CAD build for the part. Positions are in the model's coordinates, mm. A direction names the side the tool comes from. Give positions to 0.01 mm unless a question says otherwise; leave off trailing zeros. Write each loop counter-clockwise with the first axis right and the second up, starting at its lowest first coordinate (ties: lowest second). Pieces come first, ordered by that corner, then holes. Notation, with made-up numbers: (-9, 2.5) -> (11, 2.5) arc R9 ccw to (11, 7.5) -> close; hole circle Ø1 at (-7, 85.5). An arc over 180 degrees is marked (long way). Use one line per item in the form item = value. Start each with the question number.
from build123d import *

# Parameters (mm, degrees)
SKETCH1_R           = 2.5
SKETCH1_R_2         = 4
BOSS_EXTRUDE1_DEPTH = 15
SKETCH2_R           = 6.5
CUT_EXTRUDE1_DEPTH  = 8
FILLET1_R           = 7.5
CUT_EXTRUDE2_DEPTH  = 5
SKETCH5_W           = 82.5
SKETCH5_H           = 15.853105066
CUT_EXTRUDE3_DEPTH  = 15
CUT_EXTRUDE4_DEPTH  = 5
SKETCH7_R           = 2.5
BOSS_EXTRUDE2_DEPTH = 0.4


with BuildPart() as part:
    # Sketch1 → Boss-Extrude1 (new body)
    with BuildSketch(Plane(origin=(0, 0, 0), x_dir=(1, 0, 0), z_dir=(0, 1, 0))):
        Polygon((39.925742574, 57.194719472), (57.425742574, 39.694719472), (57.425742574, -162.805280528), (-42.574257426, -162.805280528), (-42.574257426, 39.694719472), (-25.074257426, 57.194719472), align=None)
        with Locations((42.175742574, 43.694719472)):
            Circle(SKETCH1_R, mode=Mode.SUBTRACT)
        with Locations((-27.324257426, 43.694719472)):
            Circle(SKETCH1_R, mode=Mode.SUBTRACT)
        with Locations((50.925742574, -36.305280528)):
            Circle(SKETCH1_R, mode=Mode.SUBTRACT)
        with Locations((-36.074257426, -36.305280528)):
            Circle(SKETCH1_R, mode=Mode.SUBTRACT)
        with Locations((50.925742574, -96.305280528)):
            Circle(SKETCH1_R, mode=Mode.SUBTRACT)
        with Locations((-36.074257426, -96.305280528)):
            Circle(SKETCH1_R, mode=Mode.SUBTRACT)
        with Locations((50.925742574, -156.305280528)):
            Circle(SKETCH1_R, mode=Mode.SUBTRACT)
        with Locations((-36.074257426, -156.305280528)):
            Circle(SKETCH1_R, mode=Mode.SUBTRACT)
        with Locations((7.425742574, -127.805280528)):
            Circle(SKETCH1_R_2, mode=Mode.SUBTRACT)
        with Locations((7.425742574, -57.805280528)):
            Circle(SKETCH1_R_2, mode=Mode.SUBTRACT)
        with Locations((7.425742574, 12.194719472)):
            Circle(SKETCH1_R_2, mode=Mode.SUBTRACT)
    extrude(amount=BOSS_EXTRUDE1_DEPTH)

    # Sketch2 → Cut-Extrude1 (cut)
    with BuildSketch(Plane(origin=(0, 15, 0), x_dir=(1, 0, 0), z_dir=(0, 1, 0))):
        with Locations((7.425742574, 12.194719472)):
            Circle(SKETCH2_R)
        with Locations((7.425742574, -57.805280528)):
            Circle(SKETCH2_R)
        with Locations((7.425742574, -127.805280528)):
            Circle(SKETCH2_R)
    extrude(amount=-CUT_EXTRUDE1_DEPTH, mode=Mode.SUBTRACT)

    # Fillet1
    fillet1_edges = [part.edges().sort_by_distance(p)[0] for p in [
        (57.425742574, 7.5, -39.694719472),
        (57.425742574, 7.5, 162.805280528),
        (-42.574257426, 7.5, 162.805280528),
        (-42.574257426, 7.5, -39.694719472),
        (-25.074257426, 7.5, -57.194719472),
        (39.925742574, 7.5, -57.194719472),
    ]]
    fillet(fillet1_edges, radius=FILLET1_R)

    # Sketch4 → Cut-Extrude2 (cut)
    with BuildSketch(Plane(origin=(0, 15, 0), x_dir=(1, 0, 0), z_dir=(0, 1, 0))):
        with BuildLine():
            Line((-26.074257426, -155.305280528), (40.925742574, -155.305280528))
            ThreePointArc((40.925742574, -155.305280528), (44.46127648, -153.840814434), (45.925742574, -150.305280528))
            Line((45.925742574, -150.305280528), (45.925742574, 34.694719472))
            ThreePointArc((45.925742574, 34.694719472), (44.46127648, 38.230253378), (40.925742574, 39.694719472))
            Line((40.925742574, 39.694719472), (-26.074257426, 39.694719472))
            ThreePointArc((-26.074257426, 39.694719472), (-29.609791332, 38.230253378), (-31.074257426, 34.694719472))
            Line((-31.074257426, 34.694719472), (-31.074257426, -150.305280528))
            ThreePointArc((-31.074257426, -150.305280528), (-29.609791332, -153.840814434), (-26.074257426, -155.305280528))
        make_face()
    extrude(amount=-CUT_EXTRUDE2_DEPTH, mode=Mode.SUBTRACT)

    # Sketch5 → Cut-Extrude3 (cut)
    with BuildSketch(Plane(origin=(0, 15, 0), x_dir=(1, 0, 0), z_dir=(0, 1, 0))):
        with Locations((7.425742574, 58.018166939)):
            Rectangle(SKETCH5_W, SKETCH5_H)
    extrude(amount=-CUT_EXTRUDE3_DEPTH, mode=Mode.SUBTRACT)

    # Sketch6 → Cut-Extrude4 (cut)
    with BuildSketch(Plane.XZ):
        Polygon((-38.441393529, 32.205280528), (-33.707121322, 32.205280528), (-31.339985218, 36.305280528), (-33.707121322, 40.405280528), (-38.441393529, 40.405280528), (-40.808529633, 36.305280528), align=None)
        Polygon((55.660014782, 36.305280528), (53.292878678, 40.405280528), (48.558606471, 40.405280528), (46.191470367, 36.305280528), (48.558606471, 32.205280528), (53.292878678, 32.205280528), align=None)
        Polygon((-22.589985218, -43.694719472), (-24.957121322, -39.594719472), (-29.691393529, -39.594719472), (-32.058529633, -43.694719472), (-29.691393529, -47.794719472), (-24.957121322, -47.794719472), align=None)
        Polygon((46.910014782, -43.694719472), (44.542878678, -39.594719472), (39.808606471, -39.594719472), (37.441470367, -43.694719472), (39.808606471, -47.794719472), (44.542878678, -47.794719472), align=None)
        Polygon((-31.339985218, 96.305280528), (-33.707121322, 100.405280528), (-38.441393529, 100.405280528), (-40.808529633, 96.305280528), (-38.441393529, 92.205280528), (-33.707121322, 92.205280528), align=None)
        Polygon((55.660014782, 96.305280528), (53.292878678, 100.405280528), (48.558606471, 100.405280528), (46.191470367, 96.305280528), (48.558606471, 92.205280528), (53.292878678, 92.205280528), align=None)
        Polygon((55.660014782, 156.305280528), (53.292878678, 160.405280528), (48.558606471, 160.405280528), (46.191470367, 156.305280528), (48.558606471, 152.205280528), (53.292878678, 152.205280528), align=None)
        Polygon((-40.808529633, 156.305280528), (-38.441393529, 152.205280528), (-33.707121322, 152.205280528), (-31.339985218, 156.305280528), (-33.707121322, 160.405280528), (-38.441393529, 160.405280528), align=None)
    extrude(amount=-CUT_EXTRUDE4_DEPTH, mode=Mode.SUBTRACT)

    # Sketch7 → Boss-Extrude2 (add)
    with BuildSketch(Plane.XZ.offset(-5)):
        with Locations((-36.074257426, 156.305280528)):
            Circle(SKETCH7_R)
        with Locations((50.925742574, 156.305280528)):
            Circle(SKETCH7_R)
        with Locations((-36.074257426, 96.305280528)):
            Circle(SKETCH7_R)
        with Locations((50.925742574, 96.305280528)):
            Circle(SKETCH7_R)
        with Locations((-36.074257426, 36.305280528)):
            Circle(SKETCH7_R)
        with Locations((50.925742574, 36.305280528)):
            Circle(SKETCH7_R)
        with Locations((-27.324257426, -43.694719472)):
            Circle(SKETCH7_R)
        with Locations((42.175742574, -43.694719472)):
            Circle(SKETCH7_R)
    extrude(amount=-BOSS_EXTRUDE2_DEPTH)


solid = part.part
1) 3-axis set-ups, long thin cutter, end or side, ignore diameter. For faces 1 (the face through (-36, 2, 152.205)), 2 (the face through (8, 13, -39.695)), 3 (the face through (9.271, 3.451, 61.354)): which of +Z, -Z, +X, -X, +Y, -Y reach the whole face in a straight line?
2) Cut at A-A (y = 12). State how many separate pieces and enclosed holes the cut face has, and give its area (3 significant figures).
3) Cut at B-B (x = 30). Give the cut face in (y, z).
4) Pin check, flat tips, straight feed: pin 1 (8 mm diameter, centred on x = 50.93, z = 156.31, fed in from +Y); pin 2 (12 mm diameter, centred on x = -23.5, z = -21, fed in from +Y); pin 3 (2.5 mm diameter, centred on x = -36.5, z = 157, fed in from +Y); pin 4 (5 mm diameter, centred on x = 50, y = 3, fed in from -Z). Stop position of each tip, or through.
5) Cut at C-C (z = 11). Give the cut face in (x, y), and give its area (4 significant figures).
6) Wall check: line 1 along X through (y, z) = (10.25, 148.5); line 2 along Z through (x, y) = (-34, 0.75); line 3 along Z through (x, y) = (-14, 13). Give the ranges that are in metal, low to high. Write a range as from..to.
7) Two-plate mould, pull along Z, no slides. Class faces 4 (the face through (8, 7, 162.805)), 5 (the face through (51, 2, 160.405)): released by +Z, released by -Z, zero draft, split by the parting line, or undercut.
Final values:
q1.face_1 = -Y
q1.face_2 = +Y
q1.face_3 = +Y, -Y
q2.separate_pieces = 1
q2.enclosed_holes = 9
q2.area = 6,000 mm^2
q3.outline = (0, -50.09) -> (15, -50.09) -> (15, -39.69) -> (10, -39.69) -> (10, 155.31) -> (15, 155.31) -> (15, 162.81) -> (0, 162.81) -> close
q4.pin_1 = 15
q4.pin_2 = 10
q4.pin_3 = 5.4
q4.pin_4 = -49.62
q5.outline = (-42.57, 0) -> (57.43, 0) -> (57.43, 15) -> (45.93, 15) -> (45.93, 10) -> (-31.07, 10) -> (-31.07, 15) -> (-42.57, 15) -> close
q5.area = 1,115 mm^2
q6.line_1 = -42.57..-31.07, 45.93..57.43
q6.line_2 = -48.27..32.21, 40.41..92.21, 100.41..152.21, 160.41..162.81
q6.line_3 = -50.09..-39.69, 155.31..162.81
q7.face_4 = released by +Z
q7.face_5 = undercut
